Could you check a few things on this drawing? It's one solid part, dimensions in mm from its lowest x, y, z. A direction names the side the tool comes from. Give positions to 0.01 mm unless a question says otherwise; leave off trailing zeros. Loops run counter-clockwise (first coordinate to the right, second up) from the corner with the lowest first, then second, coordinate; pieces in that order, holes last. Notation, with made-up numbers: M 19.5,51.5 L 59.5,51.5 A28 cw 59.5,82.5 Z; hole C -4.5,-37 d4. An arc over 180 degrees is marked long. Answer in a Markdown table with one row per item. Add a question column.
1. If we section it at B-B on y = 24: List the corners of the cut face in (x, z) for me, then the cut area to 3 significant figures.
2. I need wall thicknesses on line 1 along X through (y, z) = (14.5, 4.25); line 2 along Y through (x, z) = (5.5, 7.25); line 3 along Z through (x, y) = (7, 5.5). Which ranges of each line are inside material? Lowest first, please. Write a range as from..to.
3. I'm going to push flat-ended pins straight in: pin 1 Ø1.5 at (x, y) = (5.5, 39) entering from -Z; pin 2 Ø1.6 at (x, y) = (5, 5.5) entering from +Z. Where does each tip first touch, or does it pass through?
4. Which directions (+Z, -Z, +X, -X, +Y, -Y) give clear straight access to the entire face, cutting with the end or side of a thin tool? Please do the marked faces 1, 2 and 3.
5. If we section it at D-D on y = 7: List the corners of the cut face in (x, z) for me, then the cut area to 3 significant figures.
6. If we section it at C-C on z = 2.5: List the corners of the cut face in (x, y) for me, then the cut area to 3 significant figures.
7. If we section it at A-A on x = 4: List the corners of the cut face in (y, z) for me.
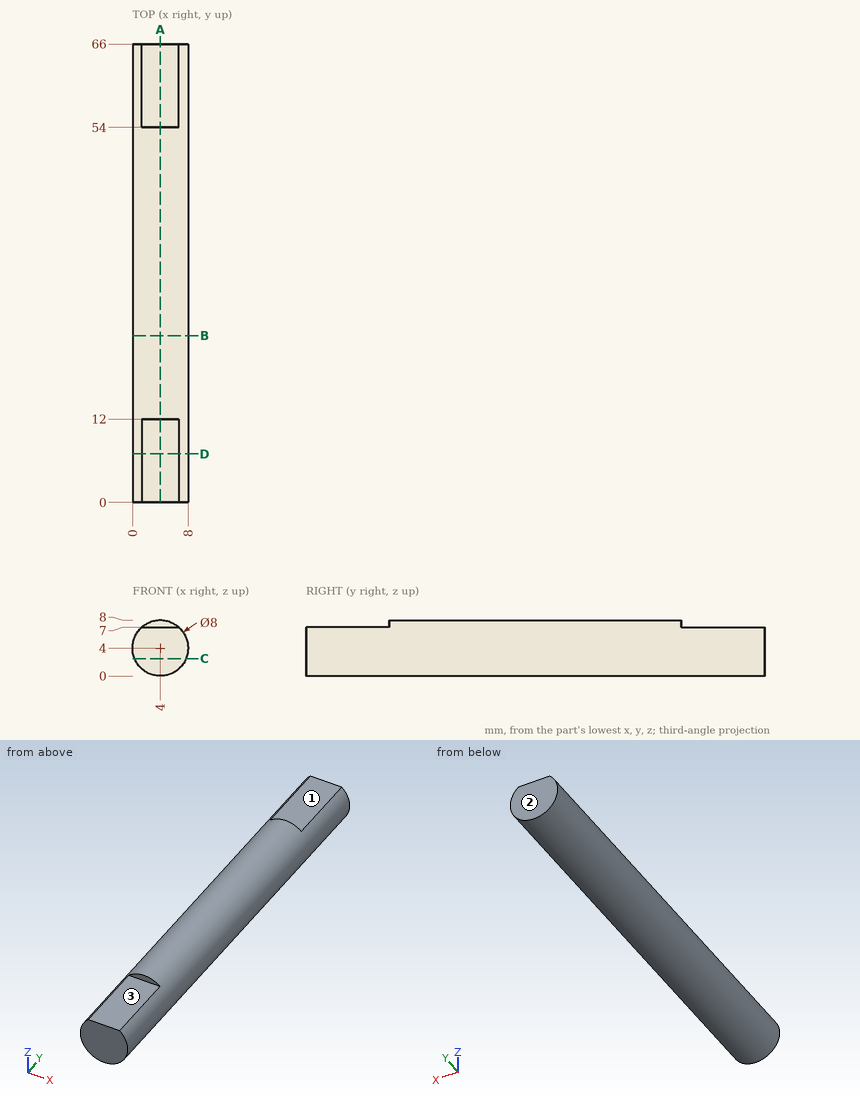
Results:
| question | item | result |
|---|---|---|
| 1 | outline | C 4,4 d8 |
| 1 | area | 50.3 mm2 |
| 2 | line 1 | 0.01..7.99 |
| 2 | line 2 | 12..54 |
| 2 | line 3 | 1.35..6.65 |
| 3 | pin 1 | z = 0.07 |
| 3 | pin 2 | z = 7 |
| 4 | face 1 | +Z, +X, -X, +Y |
| 4 | face 2 | +Z, -Z, +X, -X, +Y |
| 4 | face 3 | +Z, +X, -X, -Y |
| 5 | outline | M 1.35,7 A4 ccw long 6.65,7 Z |
| 5 | area | 46.6 mm2 |
| 6 | outline | M 0.29,0 L 7.71,0 L 7.71,66 L 0.29,66 Z |
| 6 | area | 489 mm2 |
| 7 | outline | M 0,0 L 66,0 L 66,7 L 54,7 L 54,8 L 12,8 L 12,7 L 0,7 Z |
